Work out the finished part from the listing and answer in its coordinate system (mm). Coordinates: 2 decimals unless noted, no trailing zeros. Order: outer loops, then holes, each group sorted by start corner. A loop starts at its lowest first (then second) coordinate and runs counter-clockwise, first axis right, second up. Notation, with made-up numbers: M 52.25,-18 L 110.25,-18 A20 cw 110.25,-6 Z; hole C -26.5,-13 d3. An arc over 180 degrees is marked long. Answer in a Markdown table with one row per item. Add a question column.
Item 1: Consider line 1 (Y direction, x = 22, z = -54.75); line 2 (Y direction, x = 22, z = -61.5). Determine where each line is inside the solid, lowest interval first. Write a range as from..to.
Item 2: The part is cut by section C-C (z = -65.75). Write down the section's boundary in (x, y).
Item 3: The part is cut by section A-A (y = 22). Write down the section's boundary in (x, z).
Item 4: Flat-ended cylindrical pins translate along their axes: pin 1 Ø4 at (y, z) = (23, -59) entering from +X; pin 2 Ø6 at (x, z) = (16.5, -64) entering from +Y; pin 3 Ø1.5 at (x, z) = (37.5, -63.5) entering from +Y. Find the tip coordinate at first contact, or state that the pin passes through.
Item 5: The mould has two halves that part along X. Classify faces 1 (the face through (34.932, 27.362, -54.93)), 2 (the face through (22, 25, -50)), 3 (the face through (20.16, 20.31, -59.86)): released by +X, released by -X, zero draft, split by the parting line, or undercut.
from build123d import *

# Parameters (mm, degrees)
CYLINDER004_R       = 2.5
CYLINDER004_DEPTH   = 20
CYLINDER003_R       = 14
CYLINDER003_DEPTH   = 10
CUT_PLACEMENT_ANGLE = 180


with BuildPart() as cylinder001:
    # Cylinder004 → Cylinder004 (new body)
    with BuildSketch(Plane.XY):
        Circle(CYLINDER004_R)
    extrude(amount=CYLINDER004_DEPTH)


with BuildPart() as cone:
    # Cone → Cone (revolve)
    with BuildSketch(Plane(origin=(0, 0, 10), x_dir=(1, 0, 0), z_dir=(0, -1, 0))):
        Polygon((0, 0), (14, 0), (24, 10), (0, 10), align=None)
    revolve(axis=Axis((0, 0, 10), (0, 0, 1)))


with BuildPart() as obj1:
    # Cylinder003 → Cylinder003 (new body)
    with BuildSketch(Plane.XY):
        Circle(CYLINDER003_R)
    extrude(amount=CYLINDER003_DEPTH)

    # Fusion004: union Cone
    add(cone.part)

    # Cut: cut Cylinder001
    add(cylinder001.part, mode=Mode.SUBTRACT)


with BuildPart() as obj1_1:
    # Cut placement: moved
    add(obj1.part.moved(Location((22, 22, -50))).rotate(Axis((22, 22, -50), (1, 0, 0)), CUT_PLACEMENT_ANGLE))


solid = obj1_1.part
Reply:
| question | item | result |
|---|---|---|
| 1 | line 1 | y = 8..19.5, 24.5..36 |
| 1 | line 2 | y = 6.5..19.5, 24.5..37.5 |
| 2 | outline | C 22,22 d39.5; hole C 22,22 d5 |
| 3 | outline | M -2,-70 L 19.5,-70 L 19.5,-50 L 8,-50 L 8,-60 Z; M 24.5,-70 L 46,-70 L 36,-60 L 36,-50 L 24.5,-50 Z |
| 4 | pin 1 | stops at x = 36.97 |
| 4 | pin 2 | stops at y = 42.36 |
| 4 | pin 3 | stops at y = 32.06 |
| 5 | face 1 | split by the parting line |
| 5 | face 2 | zero draft |
| 5 | face 3 | undercut |
